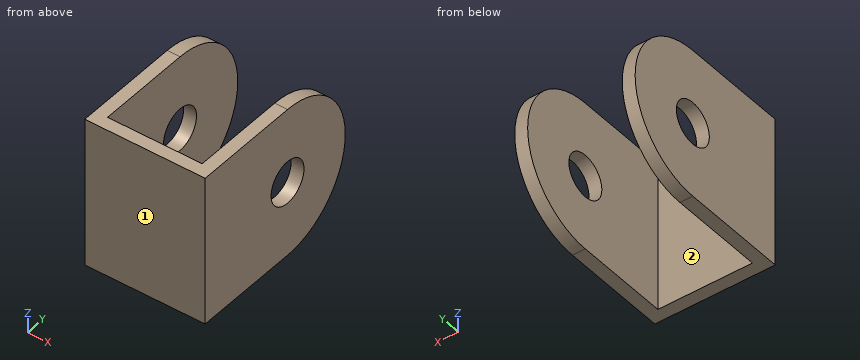
```python
from build123d import *

# Parameters (mm, degrees)
SKETCH1_W           = 22
SKETCH1_H           = 35
BOSS_EXTRUDE1_DEPTH = 3
SKETCH2_W           = 35
SKETCH2_H           = 3
BOSS_EXTRUDE6_DEPTH = 3
BOSS_EXTRUDE7_START = 3
SKETCH4_W           = 35
SKETCH4_H           = 3
BOSS_EXTRUDE7_DEPTH = 3


with BuildPart() as part:
    # Sketch1 → Boss-Extrude1 (new body)
    with BuildSketch(Plane(origin=(0, 0, 0), x_dir=(1, 0, 0), z_dir=(0, 1, 0))):
        with Locations((-45.186046512, -0.081395349)):
            Rectangle(SKETCH1_W, SKETCH1_H)
    extrude(amount=BOSS_EXTRUDE1_DEPTH)

    # Sketch2 → Boss-Extrude6 (add)
    with BuildSketch(Plane(origin=(-34.186046512, 0, 0), x_dir=(0, 0, -1), z_dir=(1, 0, 0))):
        with BuildLine():
            ThreePointArc((17.418604651, 25), (-0.081395349, 42.5), (-17.581395349, 25))
            Line((-17.581395349, 25), (-5.081395349, 25))
            ThreePointArc((-5.081395349, 25), (-0.081395349, 30), (4.918604651, 25))
            Line((4.918604651, 25), (17.418604651, 25))
        make_face()
        with BuildLine():
            Line((-5.081395349, 25), (-17.581395349, 25))
            ThreePointArc((-17.581395349, 25), (-0.081395349, 7.5), (17.418604651, 25))
            Line((17.418604651, 25), (4.918604651, 25))
            ThreePointArc((4.918604651, 25), (-0.081395349, 20), (-5.081395349, 25))
        make_face()
        with BuildLine():
            Line((-17.581395349, 25), (-17.581395349, 3))
            Line((-17.581395349, 3), (17.418604651, 3))
            Line((17.418604651, 3), (17.418604651, 25))
            ThreePointArc((17.418604651, 25), (-0.081395349, 7.5), (-17.581395349, 25))
        make_face()
        with Locations((-0.081395349, 1.5)):
            Rectangle(SKETCH2_W, SKETCH2_H)
    extrude(amount=BOSS_EXTRUDE6_DEPTH)

    # Sketch4 → Boss-Extrude7 (add)
    with BuildSketch(Plane.ZY.offset(56.186046512).offset(BOSS_EXTRUDE7_START)):
        with BuildLine():
            ThreePointArc((17.581395349, 25), (0.081395349, 42.5), (-17.418604651, 25))
            Line((-17.418604651, 25), (-4.918604651, 25))
            ThreePointArc((-4.918604651, 25), (0.081395349, 30), (5.081395349, 25))
            Line((5.081395349, 25), (17.581395349, 25))
        make_face()
        with BuildLine():
            Line((-4.918604651, 25), (-17.418604651, 25))
            ThreePointArc((-17.418604651, 25), (0.081395349, 7.5), (17.581395349, 25))
            Line((17.581395349, 25), (5.081395349, 25))
            ThreePointArc((5.081395349, 25), (0.081395349, 20), (-4.918604651, 25))
        make_face()
        with BuildLine():
            Line((-17.418604651, 25), (-17.418604651, 3))
            Line((-17.418604651, 3), (17.581395349, 3))
            Line((17.581395349, 3), (17.581395349, 25))
            ThreePointArc((17.581395349, 25), (0.081395349, 7.5), (-17.418604651, 25))
        make_face()
        with Locations((0.081395349, 1.5)):
            Rectangle(SKETCH4_W, SKETCH4_H)
    extrude(amount=-BOSS_EXTRUDE7_DEPTH)


solid = part.part
```
Can you work these out from the model? Positions are in its coordinate system, mm. Face numbers are marked on the shaded views. A direction names the side the tool comes from. Coordinates: 2 decimals unless noted, no trailing zeros. Order: outer loops, then holes, each group sorted by start corner. A loop starts at its lowest first (then second) coordinate and runs counter-clockwise, first axis right, second up. Notation, with made-up numbers: (25, 24.5) -> (39, 24.5) arc R27 ccw to (39, 54.5) -> close; hole circle Ø1 at (34, 55.5). An arc over 180 degrees is marked (long way). Write each question's results on one line, items separated by ' | '.
Item 1: I'm going to push flat-ended pins straight in: pin 1 Ø16 at (y, z) = (25, 0.08) entering from +X; pin 2 Ø5 at (x, z) = (-52, 5.5) entering from +Y; pin 3 Ø10 at (x, y) = (-45.5, 12) entering from -Z; pin 4 Ø5 at (x, z) = (-55, -8.5) entering from +Y. Where does each tip first touch, or does it pass through?
Results are:
pin 1: x = -31.19 | pin 2: y = 3 | pin 3: through | pin 4: y = 41.3
Item 2: I want a section at B-B, the plane y = 35. Write out the boundary of the cut face in (x, z).
Results are:
outline: (-59.19, -14.28) -> (-56.19, -14.28) -> (-56.19, 14.44) -> (-59.19, 14.44) -> close; (-34.19, -14.28) -> (-31.19, -14.28) -> (-31.19, 14.44) -> (-34.19, 14.44) -> close
Item 3: I want a section at D-D, the plane x = -36.25. Write out the boundary of the cut face in (y, z), then the cut area to 3 significant figures.
Results are:
outline: (0, -17.42) -> (3, -17.42) -> (3, 17.58) -> (0, 17.58) -> close | area: 105 mm²
Item 4: If I drill on line 1 along X through (y, z) = (16, 9); line 2 along Z through (x, y) = (-32.3, 25); line 3 along Y through (x, z) = (-41.5, -4.5), over which ranges is the centre line in solid material (lowest first)?
Results are:
line 1: -59.19 to -56.19, -34.19 to -31.19 | line 2: -17.42 to -4.92, 5.08 to 17.58 | line 3: 0 to 3
Item 5: Which directions (+Z, -Z, +X, -X, +Y, -Y) give clear straight access to the entire face, cutting with the end or side of a thin tool? Please do the marked faces 1 and 2.
Results are:
face 1: +Z, -Z, +X, -X, -Y | face 2: +Z, -Z, +Y
Item 6: I want a section at C-C, the plane z = 7. Write out the boundary of the cut face in (x, y).
Results are:
outline: (-59.19, 0) -> (-31.19, 0) -> (-31.19, 41.07) -> (-34.19, 41.07) -> (-34.19, 3) -> (-56.19, 3) -> (-56.19, 41.07) -> (-59.19, 41.07) -> close
Item 7: I want a section at A-A, the plane z = -3.5. Write out the boundary of the cut face in (x, y), then the cut area to 3 significant figures.
Results are:
outline: (-59.19, 0) -> (-31.19, 0) -> (-31.19, 21.51) -> (-34.19, 21.51) -> (-34.19, 3) -> (-56.19, 3) -> (-56.19, 21.51) -> (-59.19, 21.51) -> close; (-59.19, 28.49) -> (-56.19, 28.49) -> (-56.19, 42.13) -> (-59.19, 42.13) -> close; (-34.19, 28.49) -> (-31.19, 28.49) -> (-31.19, 42.13) -> (-34.19, 42.13) -> close | area: 277 mm²
